from build123d import *

# Parameters (mm, degrees)
SKETCH_1_W               = 20
SKETCH_1_H               = 45
EXTRUDE_1_DEPTH          = 12
SKETCH_2_W               = 20
SKETCH_2_H               = 20
SKETCH_2_R               = 1.5
EXTRUDE_2_DEPTH          = 6
CUT_EXTRUDE_1_DEPTH      = 57.080299571
CUT_EXTRUDE_1_DEPTH_BACK = 57.080299571
SKETCH_3_R               = 1.5
SKETCH_4_W               = 30
SKETCH_4_H               = 51
EXTRUDE_3_DEPTH          = 6
SKETCH_5_W               = 10.5
SKETCH_5_H               = 10
EXTRUDE_4_DEPTH          = 5
SKETCH_6_W               = 9
SKETCH_6_H               = 10.658350912
EXTRUDE_5_DEPTH          = 3
SKETCH_7_W               = 10.5
SKETCH_7_H               = 10
EXTRUDE_6_DEPTH          = 5
SKETCH_8_W               = 9
SKETCH_8_H               = 10.144867035
EXTRUDE_7_DEPTH          = 3
SKETCH_9_R               = 2.5
EXTRUDE_8_DEPTH          = 10
SKETCH_10_W              = 15
SKETCH_10_H              = 5
EXTRUDE_9_DEPTH          = 5
SKETCH_11_R              = 2.5
EXTRUDE_10_DEPTH         = 10
SKETCH_12_W              = 15
SKETCH_12_H              = 5
EXTRUDE_11_DEPTH         = 5


with BuildPart() as part:
    # ｽｹｯﾁ1 → ﾎﾞｽ - 押し出し1 (new body)
    with BuildSketch(Plane.XY):
        with Locations((10, 22.5)):
            Rectangle(SKETCH_1_W, SKETCH_1_H)
    extrude(amount=EXTRUDE_1_DEPTH)

    # ｽｹｯﾁ2 → ﾎﾞｽ - 押し出し2 (add)
    with BuildSketch(Plane(origin=(0, 45, 0), x_dir=(1, 0, 0), z_dir=(0, 1, 0))):
        with Locations((10, -2)):
            Rectangle(SKETCH_2_W, SKETCH_2_H)
        with Locations(Location((10, 5, 0), (0, 0, 270))):
            Circle(SKETCH_2_R, mode=Mode.SUBTRACT)
    extrude(amount=EXTRUDE_2_DEPTH)

    # ｽｹｯﾁ3 → ｶｯﾄ - 押し出し1 (cut, two sides: drawn at the far end of the back side and taken through both)
    with BuildSketch(Plane(origin=(20, 0, 0), x_dir=(0, 0, -1), z_dir=(1, 0, 0)).offset(-CUT_EXTRUDE_1_DEPTH_BACK)):
        with Locations(Location((-3, 5, 0), (0, 0, 90))):
            Circle(SKETCH_3_R)
    extrude(amount=CUT_EXTRUDE_1_DEPTH + CUT_EXTRUDE_1_DEPTH_BACK, mode=Mode.SUBTRACT)

    # ｽｹｯﾁ4 → ﾎﾞｽ - 押し出し3 (add)
    with BuildSketch(Plane.XY.offset(12)):
        with Locations((10, 25.5)):
            Rectangle(SKETCH_4_W, SKETCH_4_H)
    extrude(amount=EXTRUDE_3_DEPTH)

    # ｽｹｯﾁ5 → ﾎﾞｽ - 押し出し4 (add)
    with BuildSketch(Plane(origin=(25, 0, 0), x_dir=(0, 0, -1), z_dir=(1, 0, 0))):
        with Locations((-12.75, 15)):
            Rectangle(SKETCH_5_W, SKETCH_5_H)
    extrude(amount=EXTRUDE_4_DEPTH)

    # ｽｹｯﾁ6 → ﾎﾞｽ - 押し出し5 (add)
    with BuildSketch(Plane(origin=(0, 0, 7.5), x_dir=(-1, 0, 0), z_dir=(0, 0, -1))):
        with Locations((-25.5, 14.670824544)):
            Rectangle(SKETCH_6_W, SKETCH_6_H)
    extrude(amount=EXTRUDE_5_DEPTH)

    # ｽｹｯﾁ7 → ﾎﾞｽ - 押し出し6 (add)
    with BuildSketch(Plane.ZY.offset(5)):
        with Locations((12.75, 15)):
            Rectangle(SKETCH_7_W, SKETCH_7_H)
    extrude(amount=EXTRUDE_6_DEPTH)

    # ｽｹｯﾁ8 → ﾎﾞｽ - 押し出し7 (add)
    with BuildSketch(Plane(origin=(0, 0, 7.5), x_dir=(-1, 0, 0), z_dir=(0, 0, -1))):
        with Locations((5.5, 15.072433518)):
            Rectangle(SKETCH_8_W, SKETCH_8_H)
    extrude(amount=EXTRUDE_7_DEPTH)

    # ｽｹｯﾁ9 → ﾎﾞｽ - 押し出し8 (add)
    with BuildSketch(Plane(origin=(0, 51, 0), x_dir=(1, 0, 0), z_dir=(0, 1, 0))):
        with Locations(Location((10, 0, 0), (0, 0, 90))):
            Circle(SKETCH_9_R)
    extrude(amount=EXTRUDE_8_DEPTH)

    # ｽｹｯﾁ10 → ﾎﾞｽ - 押し出し9 (add)
    with BuildSketch(Plane(origin=(0, 61, 0), x_dir=(1, 0, 0), z_dir=(0, 1, 0))):
        with Locations((10, 0)):
            Rectangle(SKETCH_10_W, SKETCH_10_H)
    extrude(amount=-EXTRUDE_9_DEPTH)

    # ｽｹｯﾁ11 → ﾎﾞｽ - 押し出し10 (add)
    with BuildSketch(Plane.XY.offset(18)):
        with Locations((10, 21)):
            Circle(SKETCH_11_R)
    extrude(amount=EXTRUDE_10_DEPTH)

    # ｽｹｯﾁ12 → ﾎﾞｽ - 押し出し11 (add)
    with BuildSketch(Plane.XY.offset(28)):
        with Locations((10, 21)):
            Rectangle(SKETCH_12_W, SKETCH_12_H)
    extrude(amount=-EXTRUDE_11_DEPTH)


solid = part.part
Model file for the job. Use its own axes, mm. A direction names the side the tool comes from. Give positions to 0.01 mm unless a question says otherwise; leave off trailing zeros. Order: outer loops, then holes, each group sorted by start corner. A loop starts at its lowest first (then second) coordinate and runs counter-clockwise, first axis right, second up. Notation, with made-up numbers: (-18.75, 74.5) - (5.25, 74.5) arc R14 ccw to (5.25, 80.5) - close; hole circle Ø6 at (48, -28). An arc over 180 degrees is marked (long way). Write item = value, one per line. Start each with the question number.
1. Drop flat-ended pins along their axis: P1, Ø3, axis at y = 41, z = 9.5, coming from the +X side; P2, Ø5, axis at x = -4.5, z = 6, coming from the +Y side; P3, Ø4, axis at y = 21, z = 25.5, coming from the -X side; P4, Ø2.5, axis at y = 5, z = 3, coming from the -X side. Give the stop position or say it passes through.
2. Two-plate mould, pull along Y, no slides. Class faces 1 (the flat face through (5, 56, 0)), 2 (the cylindrical face through (9.86, 5.69, 1.67)), 3 (the flat face through (-6, 10, 10)), 4 (the flat face through (-7, 20, 13)): pulls with the +Y half, pulls with the -Y half, needs draft (parallel to the pull), parting line crosses it, or undercut.
3. Cut at C-C, the plane z = 5.5. List the corners of the cut face in (x, y), and give its area (3 significant figures).
4. Cut at A-A, the plane z = -5. List the corners of the cut face in (x, y).
5. Cut at D-D, the plane y = 21. List the corners of the cut face in (x, z), and give its area (3 significant figures).
6. Cut at B-B, the plane y = 5. List the corners of the cut face in (x, z), and give its area (3 significant figures).
7. Probe line 1 along X through (y, z) = (14.5, 6); line 2 along Z through (x, y) = (5, 5); line 3 along X through (y, z) = (18, 9). List the from-to ranges inside material, lowest first.
8. Which spindle directions (+Z, -Z, +X, -X, +Y, -Y) get a long thin tool onto all of the face, cutting with end or side? Do faces 5 (the flat face through (27, 10, 13)), 6 (the flat face through (25, 15, 10)), 7 (the flat face through (17.5, 59, 0)), 8 (the flat face through (2.5, 59, 0)). Say none if no direction does.
Taken from the geometry:
q1.P1 = 20
q1.P2 = 20.14
q1.P3 = 2.5
q1.P4 = through
q2.face_1 = undercut
q2.face_2 = undercut
q2.face_3 = pulls with the -Y half
q2.face_4 = pulls with the +Y half
q3.outline = (-10, 10) - (-1, 10) - (-1, 20.14) - (-10, 20.14) - close; (0, 0) - (20, 0) - (20, 51) - (0, 51) - close; (21, 9.34) - (30, 9.34) - (30, 20) - (21, 20) - close
q3.area = 1,210 mm²
q4.outline = (0, 45) - (8.5, 45) - (8.5, 51) - (0, 51) - close; (11.5, 45) - (20, 45) - (20, 51) - (11.5, 51) - close
q5.outline = (-5, 12) - (0, 12) - (0, 0) - (20, 0) - (20, 12) - (25, 12) - (25, 18) - (12.5, 18) - (12.5, 23) - (17.5, 23) - (17.5, 28) - (2.5, 28) - (2.5, 23) - (7.5, 23) - (7.5, 18) - (-5, 18) - close
q5.area = 520 mm²
q6.outline = (-5, 12) - (0, 12) - (0, 4.5) - (20, 4.5) - (20, 12) - (25, 12) - (25, 18) - (-5, 18) - close; (0, 0) - (20, 0) - (20, 1.5) - (0, 1.5) - close
q6.area = 360 mm²
q7.line_1 = -10 to -1, 0 to 20, 21 to 30
q7.line_2 = 0 to 1.5, 4.5 to 18
q7.line_3 = -10 to -5, 0 to 20, 25 to 30
q8.face_5 = +Z, +X, -Y
q8.face_6 = +Y, -Y
q8.face_7 = +Z, -Z, +X, +Y
q8.face_8 = +Z, -Z, -X, +Y
